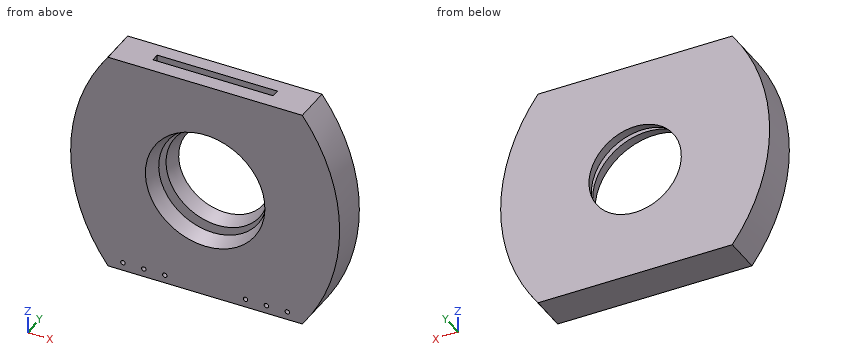
```python
from build123d import *

# Parameters (mm, degrees)
BOSS_EXTRUDE1_DEPTH  = 50
CARBON_FILTER_HOLE_W = 161
CARBON_FILTER_HOLE_H = 11
CUT_EXTRUDE3_DEPTH   = 280
SKETCH1_R            = 3
CUT_EXTRUDE4_DEPTH   = 20


with BuildPart() as part:
    # Lid case → Boss-Extrude1 (new body)
    with BuildSketch(Plane(origin=(0, 0, 0), x_dir=(1, 0, 0), z_dir=(0, 1, 0))):
        with BuildLine():
            Line((-130, 150), (130, 150))
            ThreePointArc((130, 150), (180, 0), (130, -150))
            Line((130, -150), (-130, -150))
            ThreePointArc((-130, -150), (-180, 0), (-130, 150))
        make_face()
    extrude(amount=BOSS_EXTRUDE1_DEPTH)

    # Ventilation → Cut-Revolve1 (revolve, cut)
    with BuildSketch(Plane.XY, mode=Mode.PRIVATE) as cut_revolve1_sk:
        Polygon((0, 50), (0, 0), (-80, 0), (-61.801488287, 50), align=None)
    revolve(cut_revolve1_sk.sketch.rotate(Axis((0, -54.373231572, 0), (0, 1, 0)), 270), axis=Axis((0, -54.373231572, 0), (0, 1, 0)), mode=Mode.SUBTRACT)

    # Carbon filter hole → Cut-Extrude3 (cut)
    with BuildSketch(Plane.XY.offset(150)):
        with Locations((0, 25.5)):
            Rectangle(CARBON_FILTER_HOLE_W, CARBON_FILTER_HOLE_H)
    extrude(amount=-CUT_EXTRUDE3_DEPTH, mode=Mode.SUBTRACT)

    # Sketch1 → Cut-Extrude4 (cut)
    with BuildSketch(Plane.XZ):
        with Locations(Location((-110, -139, 0), (0, 0, 270))):
            Circle(SKETCH1_R)
        with Locations(Location((-82, -139, 0), (0, 0, 270))):
            Circle(SKETCH1_R)
        with Locations(Location((-54, -139, 0), (0, 0, 270))):
            Circle(SKETCH1_R)
        with Locations(Location((54, -139, 0), (0, 0, 270))):
            Circle(SKETCH1_R)
        with Locations(Location((82, -139, 0), (0, 0, 270))):
            Circle(SKETCH1_R)
        with Locations(Location((110, -139, 0), (0, 0, 270))):
            Circle(SKETCH1_R)
    extrude(amount=-CUT_EXTRUDE4_DEPTH, mode=Mode.SUBTRACT)


solid = part.part
```
Verification items for the finished model (mm, model axes). Coordinates: 2 decimals unless noted, no trailing zeros. Loops run counter-clockwise (first coordinate to the right, second up) from the corner with the lowest first, then second, coordinate; pieces in that order, holes last. Notation, with made-up numbers: (62.5, -20) -> (66.5, -20) arc R16 cw to (66.5, -10) -> close; hole circle Ø7 at (-16.75, 7). An arc over 180 degrees is marked (long way). Answer in a Markdown table with one row per item.
1) Section check C-C (z = -90.5). Record the cut outline in (x, y).
The answers:
| item | result |
|---|---|
| outline | (-163.04, 0) -> (163.04, 0) -> (163.04, 50) -> (-163.04, 50) -> close; hole (-80.5, 20) -> (80.5, 20) -> (80.5, 31) -> (-80.5, 31) -> close |
2) Section check A-A (x = 0). Record the cut outline in (y, z), and give its area (3 significant figures).
The answers:
| item | result |
|---|---|
| outline | (0, -150) -> (50, -150) -> (50, -61.8) -> (31, -68.72) -> (31, -130) -> (20, -130) -> (20, -72.72) -> (0, -80) -> close; (0, 80) -> (20, 72.72) -> (20, 150) -> (0, 150) -> close; (31, 68.72) -> (50, 61.8) -> (50, 150) -> (31, 150) -> close |
| area | 6,390 mm2 |
3) Scan lines: line 1 along Y through (x, z) = (57.5, 105.5); line 2 along X through (y, z) = (33, -43); line 3 along Z through (x, y) = (56.5, 16). Record each from-to range of solid material in increasing order. Write a range as from..to.
The answers:
| item | result |
|---|---|
| line 1 | y = 0..20, 31..50 |
| line 2 | x = -176.27..-52.66, 52.66..176.27 |
| line 3 | z = -150..-140.66, -137.34..-48.06, 48.06..150 |
4) Section check B-B (y = 13). Record the cut outline in (x, z).
The answers:
| item | result |
|---|---|
| outline | (-130, -150) -> (130, -150) arc R250 ccw to (130, 150) -> (-130, 150) arc R250 ccw to start; hole circle Ø6 at (-110, -139); hole circle Ø6 at (-82, -139); hole circle Ø150.54 at (0, 0); hole circle Ø6 at (-54, -139); hole circle Ø6 at (54, -139); hole circle Ø6 at (82, -139); hole circle Ø6 at (110, -139) |
5) Depth check by flat-ended pin: P1, Ø5, axis at x = 108.5, z = -138.5, coming from the -Y side; P2, Ø9, axis at y = 26, z = 48, coming from the +X side; P3, Ø3, axis at y = 17, z = -95, coming from the -X side; P4, Ø8, axis at x = 42, y = 25, coming from the +Z side. Enter the tip coordinate at first touch or a pass-through.
The answers:
| item | result |
|---|---|
| P1 | stops at y = 0 |
| P2 | stops at x = 176.19 |
| P3 | stops at x = -161.86 |
| P4 | stops at z = -130 |
6) Section check D-D (y = 42). Record the cut outline in (x, z).
The answers:
| item | result |
|---|---|
| outline | (-130, -150) -> (130, -150) arc R250 ccw to (130, 150) -> (-130, 150) arc R250 ccw to start; hole circle Ø129.43 at (0, 0) |
